Drawing for the job (mm, zero at the part's lowest x, y, z). A direction names the side the tool comes from. Coordinates: 2 decimals unless noted, no trailing zeros. Order: outer loops, then holes, each group sorted by start corner. A loop starts at its lowest first (then second) coordinate and runs counter-clockwise, first axis right, second up.
1) Cut at C-C (x = 10.5). List the corners of the cut face in (y, z).
2) Wall check: L1, parallel to Y at x = 17, z = 2; L2, parallel to Y at x = 16.25, z = 4; L3, parallel to Z at x = 16.5, y = 6.5. Give the ranges that are in metal, low to high.
3) Mould opens along X. For the marked faces 3, 4, 5 and 6 say: +X half, -X half, draft (parallel to the pull), parting line (faces both ways), or undercut.
4) Tool access for the marked faces 1 and 2: list every direction of +Z, -Z, +X, -X, +Y, -Y with a clear straight run to the whole face (end or side of a thin tool).
5) Cut at D-D (x = 17). List the corners of the cut face in (y, z), and give its area (3 significant figures).
6) Pin check, flat tip, straight feed: pin 1 Ø3 at (y, z) = (24, 3.5) entering from +X. Stop position of the tip, or through.
7) Cut at B-B (z = 1.75). List the corners of the cut face in (x, y), and give its area (3 significant figures).
8) Cut at A-A (y = 3). List the corners of the cut face in (x, z), and give its area (3 significant figures).
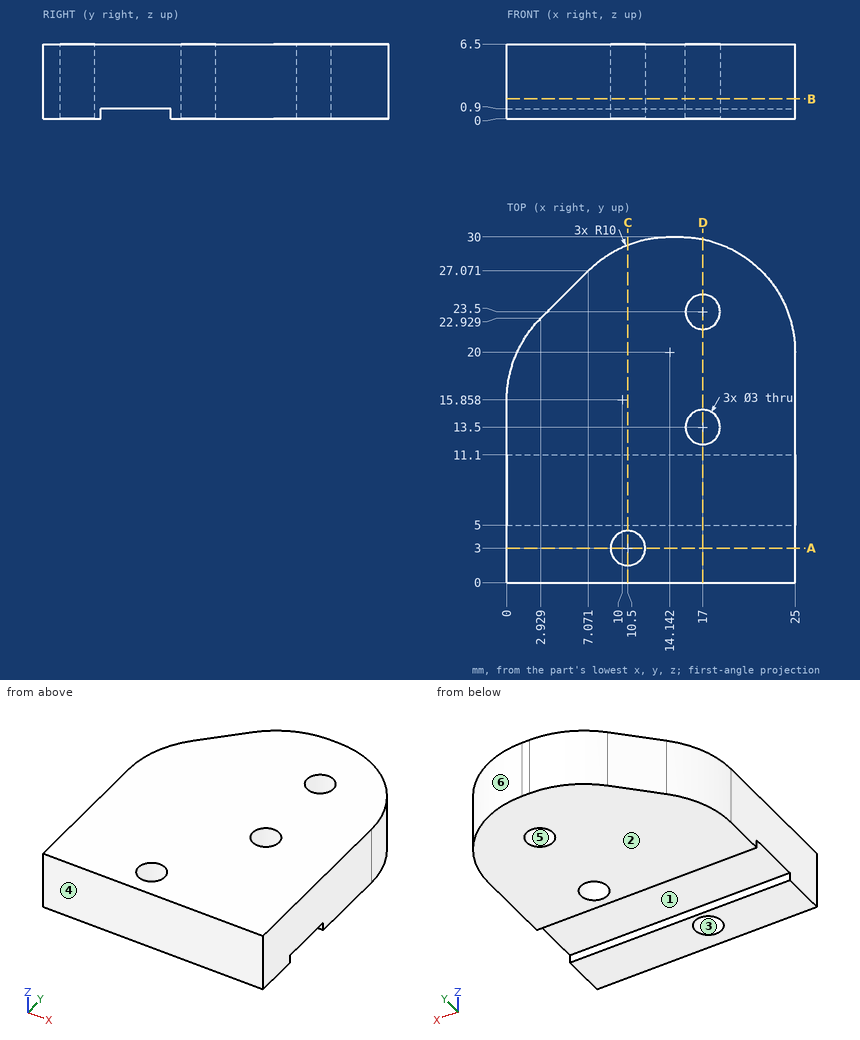
Geometry check:
1. outline: (0, 0) - (1.5, 0) - (1.5, 6.5) - (0, 6.5) - close; (4.5, 0) - (5, 0) - (5, 0.9) - (11.1, 0.9) - (11.1, 0) - (29.31, 0) - (29.31, 6.5) - (4.5, 6.5) - close
2. L1: y = 0 to 12, 15 to 22, 25 to 29.8
2. L2: y = 0 to 12.2, 14.8 to 22.2, 24.8 to 29.92
2. L3: z = 0.9 to 6.5
3. face 3: undercut
3. face 4: draft
3. face 5: undercut
3. face 6: +X half
4. face 1: -Z, +X, -X
4. face 2: -Z, +X, -X, +Y, -Y
5. outline: (0, 0) - (5, 0) - (5, 0.9) - (11.1, 0.9) - (11.1, 0) - (12, 0) - (12, 6.5) - (0, 6.5) - close; (15, 0) - (22, 0) - (22, 6.5) - (15, 6.5) - close; (25, 0) - (29.8, 0) - (29.8, 6.5) - (25, 6.5) - close
5. area: 149 mm2
6. pin 1: stops at x = 24.68
7. outline: (0, 0) - (25, 0) - (25, 20) arc R10 ccw to (15, 30) - (14.14, 30) arc R10 ccw to (7.07, 27.07) - (2.93, 22.93) arc R10 ccw to (0, 15.86) - close; hole circle Ø3 at (10.5, 3); hole circle Ø3 at (17, 13.5); hole circle Ø3 at (17, 23.5)
7. area: 653 mm2
8. outline: (0, 0) - (9, 0) - (9, 6.5) - (0, 6.5) - close; (12, 0) - (25, 0) - (25, 6.5) - (12, 6.5) - close
8. area: 143 mm2
